For this review, take the finished solid that the model builds, in its own axes (mm). Face numbers are marked on the shaded views. A direction names the side the tool comes from. Give positions to 0.01 mm unless a question says otherwise; leave off trailing zeros. Loops run counter-clockwise (first coordinate to the right, second up) from the corner with the lowest first, then second, coordinate; pieces in that order, holes last.
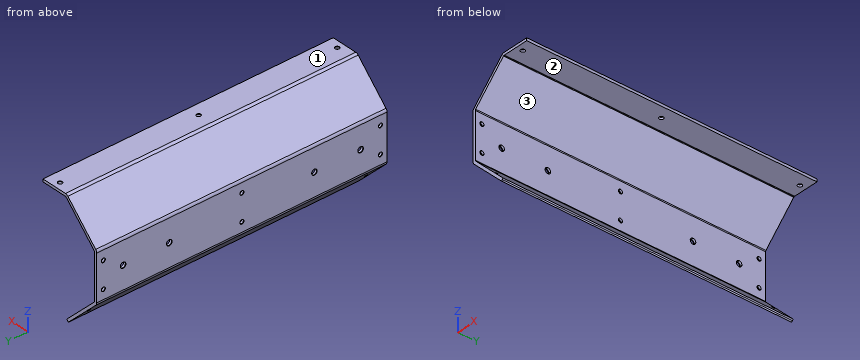
```python
from build123d import *
from build123d.topology import SkipClean

# Parameters (mm, degrees)
EXTRUDE_1_DEPTH             = 220
SKETCH_3_R                  = 1.55
SKETCH_3_R_2                = 2.1
CUT_EXTRUDE_1_DEPTH         = 10
SKETCH_6_R                  = 1.6
CUT_EXTRUDE_2_DEPTH         = 10
CHAMFER_1_SIZE              = 1
CHAMFER_1_SIZE2             = 0.707106781
SHEET_START                 = -114.419250373
SHEET_METAL_2_OUTLINE_W     = 220
SHEET_METAL_2_OUTLINE_H     = 86.5
SHEET_METAL_2_OUTLINE_R     = 1.55
SHEET_METAL_2_OUTLINE_R_2   = 2.1
SHEET_METAL_2_DEPTH         = 26.274603255
SHEET_START_2               = -87.816219993
SHEET_METAL_2_2_OUTLINE_W   = 220
SHEET_METAL_2_2_OUTLINE_H   = 87
SHEET_METAL_2_2_OUTLINE_R   = 1.55
SHEET_METAL_2_2_OUTLINE_R_2 = 2.1
SHEET_METAL_2_2_DEPTH       = 0.483052927
SHEET_START_3               = -89.230433555
SHEET_METAL_2_3_OUTLINE_W   = 220
SHEET_METAL_2_3_OUTLINE_H   = 0.5
SHEET_METAL_2_3_DEPTH       = 21.707106781
SHEET_METAL_2_4_DEPTH       = 220
SHEET_METAL_2_5_DEPTH       = 220
SHEET_START_4               = 44
SHEET_METAL_2_6_OUTLINE_R   = 1.6
SHEET_METAL_2_6_DEPTH       = 0.5
SKETCH_7_R                  = 1.5
CUT_EXTRUDE_3_DEPTH         = 10


with BuildPart() as part:
    # 草图2 → 凸台-拉伸1 (new body)
    with BuildSketch(Plane(origin=(0, 0, 0), x_dir=(1, 0, 0), z_dir=(0, 1, 0))):
        Polygon((-87.523326774, 42.5), (-112.419250373, 17.604076401), (-112.419250373, -17.604076401), (-87.523326774, -42.5), (-67.523326774, -42.5), (-67.523326774, -44), (-88.144647118, -44), (-113.919250373, -18.225396744), (-113.919250373, 18.225396744), (-89.644647118, 42.5), align=None)
    extrude(amount=EXTRUDE_1_DEPTH)

    # Sketch 3 → 切除-拉伸1 (cut)
    with BuildSketch(Plane.ZY.offset(113.919250373)):
        with Locations((-10, 5)):
            Circle(SKETCH_3_R)
        with Locations((10, 5)):
            Circle(SKETCH_3_R)
        with BuildLine():
            ThreePointArc((-8.45, 110), (-10, 111.55), (-11.55, 110))
            Line((-11.55, 110), (-8.45, 110))
        make_face()
        with BuildLine():
            Line((-8.45, 110), (-11.55, 110))
            ThreePointArc((-11.55, 110), (-10, 108.45), (-8.45, 110))
        make_face()
        with BuildLine():
            ThreePointArc((8.45, 110), (10, 108.45), (11.55, 110))
            Line((11.55, 110), (8.45, 110))
        make_face()
        with BuildLine():
            Line((8.45, 110), (11.55, 110))
            ThreePointArc((11.55, 110), (10, 111.55), (8.45, 110))
        make_face()
        with Locations((-10, 215)):
            Circle(SKETCH_3_R)
        with Locations((10, 215)):
            Circle(SKETCH_3_R)
        with Locations((0, 200)):
            Circle(SKETCH_3_R_2)
        with Locations((0, 165)):
            Circle(SKETCH_3_R_2)
        with Locations((0, 55)):
            Circle(SKETCH_3_R_2)
        with Locations((0, 20)):
            Circle(SKETCH_3_R_2)
    extrude(amount=-CUT_EXTRUDE_1_DEPTH, mode=Mode.SUBTRACT)

    # 草图6 → 切除-拉伸2 (cut)
    with BuildSketch(Plane.XY.offset(44)):
        with Locations((-76.693326774, 5)):
            Circle(SKETCH_6_R)
        with Locations((-76.693326774, 110)):
            Circle(SKETCH_6_R)
        with Locations((-76.693326774, 215)):
            Circle(SKETCH_6_R)
    extrude(amount=-CUT_EXTRUDE_2_DEPTH, mode=Mode.SUBTRACT)

    # 倒角1
    chamfer_1_edges = [part.edges().sort_by_distance(p)[0] for p in [
        (-87.523326774, 110, -42.5),
    ]]
    chamfer_1_side = [part.faces().sort_by_distance(p)[0] for p in [
        (-99.971288574, 110, -30.0520382),
    ]]
    chamfer(chamfer_1_edges, length=CHAMFER_1_SIZE, length2=CHAMFER_1_SIZE2, reference=chamfer_1_side[0])

    # Sheet Metal 2: read off the stored shape, not the designer's step
    # Sheet Metal 2 outline → Sheet Metal 2 (add)
    with SkipClean():  # the faces are left unmerged after this step: merging them gives an invalid solid
        with BuildSketch(Plane.YZ.offset(SHEET_START)):
            with Locations((110, 0.75)):
                Rectangle(SHEET_METAL_2_OUTLINE_W, SHEET_METAL_2_OUTLINE_H)
            with Locations((5, -10)):
                Circle(SHEET_METAL_2_OUTLINE_R, mode=Mode.SUBTRACT)
            with Locations((20, 0)):
                Circle(SHEET_METAL_2_OUTLINE_R_2, mode=Mode.SUBTRACT)
            with Locations((55, 0)):
                Circle(SHEET_METAL_2_OUTLINE_R_2, mode=Mode.SUBTRACT)
            with Locations((110, -10)):
                Circle(SHEET_METAL_2_OUTLINE_R, mode=Mode.SUBTRACT)
            with Locations((215, -10)):
                Circle(SHEET_METAL_2_OUTLINE_R, mode=Mode.SUBTRACT)
            with Locations((165, 0)):
                Circle(SHEET_METAL_2_OUTLINE_R_2, mode=Mode.SUBTRACT)
            with Locations((200, 0)):
                Circle(SHEET_METAL_2_OUTLINE_R_2, mode=Mode.SUBTRACT)
            with Locations((5, 10)):
                Circle(SHEET_METAL_2_OUTLINE_R, mode=Mode.SUBTRACT)
            with Locations((110, 10)):
                Circle(SHEET_METAL_2_OUTLINE_R, mode=Mode.SUBTRACT)
            with Locations((215, 10)):
                Circle(SHEET_METAL_2_OUTLINE_R, mode=Mode.SUBTRACT)
        extrude(amount=SHEET_METAL_2_DEPTH)

    # Sheet Metal 2 2 outline → Sheet Metal 2 2 (add)
    with SkipClean():  # the faces are left unmerged after this step: merging them gives an invalid solid
        with BuildSketch(Plane.YZ.offset(SHEET_START_2)):
            with Locations((110, 1)):
                Rectangle(SHEET_METAL_2_2_OUTLINE_W, SHEET_METAL_2_2_OUTLINE_H)
            with Locations((5, -10)):
                Circle(SHEET_METAL_2_2_OUTLINE_R, mode=Mode.SUBTRACT)
            with Locations((20, 0)):
                Circle(SHEET_METAL_2_2_OUTLINE_R_2, mode=Mode.SUBTRACT)
            with Locations((55, 0)):
                Circle(SHEET_METAL_2_2_OUTLINE_R_2, mode=Mode.SUBTRACT)
            with Locations((110, -10)):
                Circle(SHEET_METAL_2_2_OUTLINE_R, mode=Mode.SUBTRACT)
            with Locations((215, -10)):
                Circle(SHEET_METAL_2_2_OUTLINE_R, mode=Mode.SUBTRACT)
            with Locations((165, 0)):
                Circle(SHEET_METAL_2_2_OUTLINE_R_2, mode=Mode.SUBTRACT)
            with Locations((200, 0)):
                Circle(SHEET_METAL_2_2_OUTLINE_R_2, mode=Mode.SUBTRACT)
            with Locations((5, 10)):
                Circle(SHEET_METAL_2_2_OUTLINE_R, mode=Mode.SUBTRACT)
            with Locations((110, 10)):
                Circle(SHEET_METAL_2_2_OUTLINE_R, mode=Mode.SUBTRACT)
            with Locations((215, 10)):
                Circle(SHEET_METAL_2_2_OUTLINE_R, mode=Mode.SUBTRACT)
        extrude(amount=SHEET_METAL_2_2_DEPTH)

    # Sheet Metal 2 3 outline → Sheet Metal 2 3 (add)
    with SkipClean():  # the faces are left unmerged after this step: merging them gives an invalid solid
        with BuildSketch(Plane.YZ.offset(SHEET_START_3)):
            with Locations((110, 44.25)):
                Rectangle(SHEET_METAL_2_3_OUTLINE_W, SHEET_METAL_2_3_OUTLINE_H)
        extrude(amount=SHEET_METAL_2_3_DEPTH)

    # Sheet Metal 2 4 outline → Sheet Metal 2 4 (cut)
    with BuildSketch(Plane(origin=(0, 0, 0), x_dir=(1, 0, 0), z_dir=(0, 1, 0))):
        with BuildLine():
            Line((-87.816219993, 42.5), (-87.816219993, -42.207106781))
            ThreePointArc((-87.816219993, -42.207106781), (-87.593520149, -42.374842797), (-87.333167066, -42.474576765))
            Line((-87.333167066, -42.474576765), (-87.333167066, 42.5))
            Line((-87.333167066, 42.5), (-87.816219993, 42.5))
        make_face()
        with BuildLine():
            Line((-88.144647118, 42.5), (-88.937540337, 42.5))
            Line((-88.937540337, 42.5), (-88.230433555, 41.792893219))
            Line((-88.230433555, 41.792893219), (-112.126357154, 17.89696962))
            ThreePointArc((-112.126357154, 17.89696962), (-112.343129906, 17.572546271), (-112.419250373, 17.189862838))
            Line((-112.419250373, 17.189862838), (-112.419250373, -17.189862838))
            ThreePointArc((-112.419250373, -17.189862838), (-112.343129906, -17.572546271), (-112.126357154, -17.89696962))
            Line((-112.126357154, -17.89696962), (-88.144647118, -41.878679656))
            Line((-88.144647118, -41.878679656), (-88.144647118, 42.5))
        make_face()
        with BuildLine():
            ThreePointArc((-113.540570717, -19.311183182), (-114.190888971, -18.337913135), (-114.419250373, -17.189862838))
            Line((-114.419250373, -17.189862838), (-114.419250373, -44))
            Line((-114.419250373, -44), (-89.230433555, -44))
            Line((-89.230433555, -44), (-89.230433555, -44.5))
            Line((-89.230433555, -44.5), (-87.109113212, -44.5))
            ThreePointArc((-87.109113212, -44.5), (-88.257163509, -44.271638598), (-89.230433555, -43.621320344))
            Line((-89.230433555, -43.621320344), (-113.540570717, -19.311183182))
        make_face()
        with BuildLine():
            Line((-113.540570717, 19.311183182), (-90.351753899, 42.5))
            Line((-90.351753899, 42.5), (-114.419250373, 42.5))
            Line((-114.419250373, 42.5), (-114.419250373, 17.189862838))
            ThreePointArc((-114.419250373, 17.189862838), (-114.190888971, 18.337913135), (-113.540570717, 19.311183182))
        make_face()
    extrude(amount=SHEET_METAL_2_4_DEPTH, mode=Mode.SUBTRACT)

    # Sheet Metal 2 5 outline → Sheet Metal 2 5 (add)
    with BuildSketch(Plane(origin=(0, 0, 0), x_dir=(1, 0, 0), z_dir=(0, 1, 0))):
        with BuildLine():
            ThreePointArc((-87.109113212, -42.5), (-87.221859022, -42.493623864), (-87.333167066, -42.474576765))
            Line((-87.333167066, -42.474576765), (-87.333167066, -42.5))
            Line((-87.333167066, -42.5), (-87.109113212, -42.5))
        make_face()
        Polygon((-88.937540337, 42.5), (-89.644647118, 43.207106781), (-90.351753899, 42.5), align=None)
    extrude(amount=SHEET_METAL_2_5_DEPTH)

    # Sheet Metal 2 6 outline → Sheet Metal 2 6 (cut)
    with BuildSketch(Plane.XY.offset(SHEET_START_4)):
        with Locations((-76.693326774, 5)):
            Circle(SHEET_METAL_2_6_OUTLINE_R)
        with Locations((-76.693326774, 110)):
            Circle(SHEET_METAL_2_6_OUTLINE_R)
        with Locations((-76.693326774, 215)):
            Circle(SHEET_METAL_2_6_OUTLINE_R)
    extrude(amount=SHEET_METAL_2_6_DEPTH, mode=Mode.SUBTRACT)

    # 草图7 → 切除-拉伸3 (cut)
    with BuildSketch(Plane(origin=(-66.425876949, 0, -66.425876949), x_dir=(-0.7071067811865474, 0, 0.7071067811865477), z_dir=(-0.7071067811865477, 0, -0.7071067811865474))):
        with Locations((49.436299673, 215)):
            Circle(SKETCH_7_R)
        with Locations((49.436299673, 5)):
            Circle(SKETCH_7_R)
    extrude(amount=-CUT_EXTRUDE_3_DEPTH, mode=Mode.SUBTRACT)


solid = part.part
```
Q1. For pin 1 Ø3.5 at (y, z) = (5, -10) entering from +X; pin 2 Ø6 at (x, y) = (-81.5, 164.5) entering from -Z; pin 3 Ø12 at (y, z) = (57, 25) entering from +X; pin 4 Ø3.5 at (y, z) = (20, 0) entering from +X, all flat-tipped, find the tip position at first contact; note any pin that passes through.
Answers:
pin 1: stops at x = -112.42
pin 2: stops at z = 42.5
pin 3: stops at x = -99.02
pin 4: passes through
Q2. Consider section A-A on y = 41. Give the boundary of the cut face in (x, z), plus the area to 3 significant figures.
Answers:
outline: (-114.42, -17.19) arc R3 ccw to (-113.54, -19.31) - (-89.64, -43.21) - (-88.23, -41.79) - (-112.13, -17.9) arc R1 cw to (-112.42, -17.19) - (-112.42, 17.19) arc R1 cw to (-112.13, 17.9) - (-87.82, 42.21) arc R1 cw to (-87.11, 42.5) - (-67.52, 42.5) - (-67.52, 44.5) - (-87.11, 44.5) arc R3 ccw to (-89.23, 43.62) - (-113.54, 19.31) arc R3 ccw to (-114.42, 17.19) - close
area: 254 mm2
Q3. Consider section C-C on x = -81.5. Give the boundary of the cut face in (y, z).
Answers:
outline: (0, 42.5) - (220, 42.5) - (220, 44.5) - (0, 44.5) - close
Q4. Consider section B-B on z = -4.5. Give the boundary of the cut face in (x, y).
Answers:
outline: (-114.42, 0) - (-112.42, 0) - (-112.42, 220) - (-114.42, 220) - close
Q5. For probe 1 along Y at (x, z) = (-113.3, 0); probe 2 along Y at (x, z) = (-114.2, -10); probe 3 along Z at (x, y) = (-78, 88.5), list the stretches that pass through material, from the lowest coordinate up.
Answers:
probe 1: y = 0 to 17.9, 22.1 to 52.9, 57.1 to 162.9, 167.1 to 197.9, 202.1 to 220
probe 2: y = 0 to 3.45, 6.55 to 108.45, 111.55 to 213.45, 216.55 to 220
probe 3: z = 42.5 to 44.5
Q6. Machinability: for the marked faces 1, 2 and 3, which of the approach directions +Z, -Z, +X, -X, +Y, -Y give a long, thin tool a straight path to every point of the face, cutting with its end or side? Answer none if there is none.
Answers:
face 1: +Z, +X, -X, +Y, -Y
face 2: -Z, +X, +Y, -Y
face 3: +X, +Y, -Y
